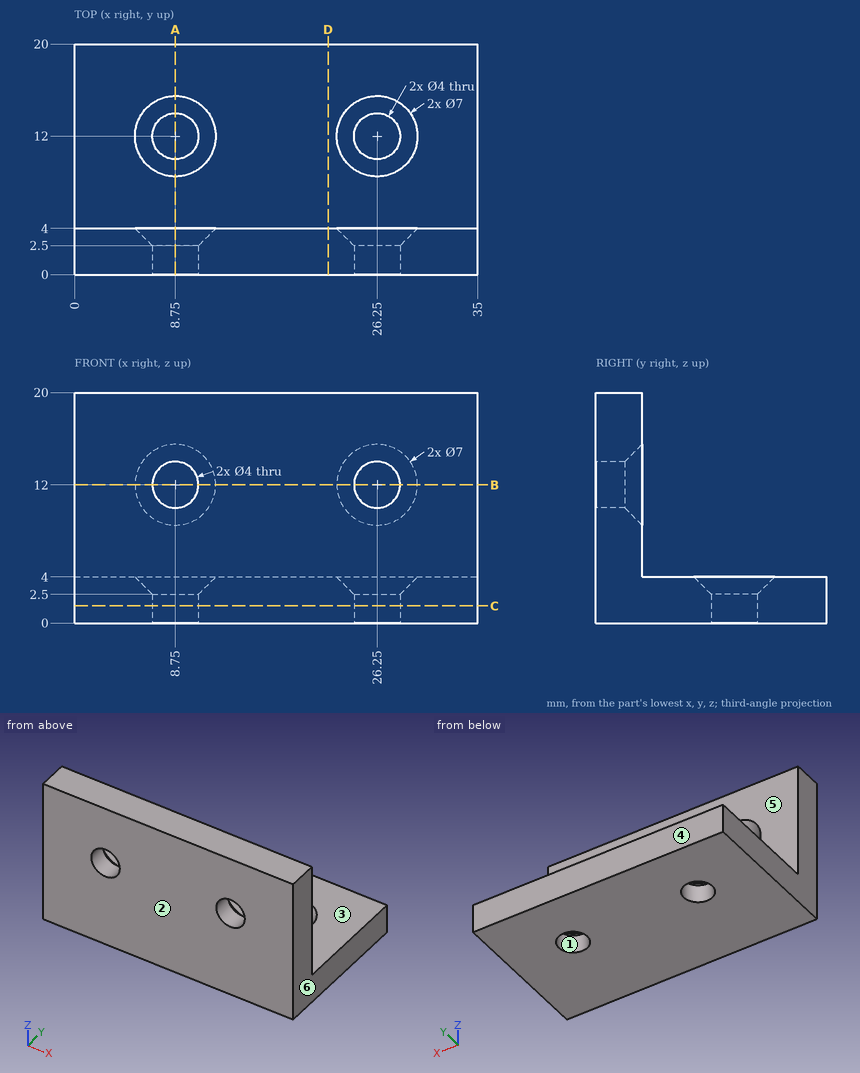
Design review of the part shown in the three views and the two pictorial views. Dimensions are in mm from the part's minimum x, y and z. A direction names the side the tool comes from. Give positions to 0.01 mm unless a question says otherwise; leave off trailing zeros. Loops run counter-clockwise (first coordinate to the right, second up) from the corner with the lowest first, then second, coordinate; pieces in that order, holes last. Notation, with made-up numbers: (64.25, 59.25) -> (94.25, 59.25) arc R17 ccw to (94.25, 71.25) -> close; hole circle Ø4 at (-2.75, 1). An arc over 180 degrees is marked (long way). Put each result on its own line as item: value. Start each with the question number.
1. For the marked faces 5 and 6, list the 3-axis set-ups (+Z, -Z, +X, -X, +Y, -Y) from which the entire face can be reached by the end or side of a thin tool; tool diameter is ignored.
2. We need section B-B on z = 12. State the section outline as (x, y) points.
3. Wall thickness on probe 1 along X at (y, z) = (1.3, 12); probe 2 along Y at (x, z) = (26.25, 1.5): over which ranges is each line inside the solid? List them lowest first.
4. Clearance check with flat-ended pins moving along their axes: P1, Ø5, axis at x = 19.5, z = 12.5, coming from the +Y side; P2, Ø2, axis at x = 17.5, y = 15, coming from the +Z side; P3, Ø4.5, axis at x = 26.25, y = 12, coming from the +Z side. State where each tip first meets the part, or that it passes through.
5. We need section A-A on x = 8.75. State the section outline as (y, z) points.
6. We need section D-D on x = 22. State the section outline as (y, z) points, then the cut area to 3 significant figures.
7. Mouldability with a two-part tool opening along Y and no side actions: class the marked faces 1, 2, 3 and 4 as released by +Y, released by -Y, zero draft, split by the parting line, or undercut.
8. We need section C-C on z = 1.5. State the section outline as (x, y) points.
Determined:
1. face 5: +Z, +X, -X, +Y
1. face 6: +Z, -Z, +X, +Y, -Y
2. outline: (0, 0) -> (6.75, 0) -> (6.75, 2.5) -> (5.25, 4) -> (0, 4) -> close; (10.75, 0) -> (24.25, 0) -> (24.25, 2.5) -> (22.75, 4) -> (12.25, 4) -> (10.75, 2.5) -> close; (28.25, 0) -> (35, 0) -> (35, 4) -> (29.75, 4) -> (28.25, 2.5) -> close
3. probe 1: 0 to 6.75, 10.75 to 24.25, 28.25 to 35
3. probe 2: 0 to 10, 14 to 20
4. P1: y = 4
4. P2: z = 4
4. P3: z = 2.75
5. outline: (0, 0) -> (10, 0) -> (10, 2.5) -> (8.5, 4) -> (4, 4) -> (4, 8.5) -> (2.5, 10) -> (0, 10) -> close; (0, 14) -> (2.5, 14) -> (4, 15.5) -> (4, 20) -> (0, 20) -> close; (14, 0) -> (20, 0) -> (20, 4) -> (15.5, 4) -> (14, 2.5) -> close
6. outline: (0, 0) -> (20, 0) -> (20, 4) -> (4, 4) -> (4, 20) -> (0, 20) -> close
6. area: 144 mm^2
7. face 1: undercut
7. face 2: released by -Y
7. face 3: zero draft
7. face 4: released by +Y
8. outline: (0, 0) -> (35, 0) -> (35, 20) -> (0, 20) -> close; hole circle Ø4 at (8.75, 12); hole circle Ø4 at (26.25, 12)
